from build123d import *

# Parameters (mm, degrees)
SKETCH1_R           = 6
BOSS_EXTRUDE1_DEPTH = 10
BOSS_EXTRUDE1_TAPER = 15
SKETCH2_R           = 2
CUT_EXTRUDE1_DEPTH  = 14.114877049
SKETCH3_W           = 4.267949192
SKETCH3_H           = 2
CUT_EXTRUDE2_DEPTH  = 14.114877049


with BuildPart() as part:
    # Sketch1 → Boss-Extrude1 (new body)
    with BuildSketch(Plane.XY):
        Circle(SKETCH1_R)
    extrude(amount=BOSS_EXTRUDE1_DEPTH, taper=BOSS_EXTRUDE1_TAPER)

    # Sketch2 → Cut-Extrude1 (cut, through all)
    with BuildSketch(Plane(origin=(0, 0, 0), x_dir=(-1, 0, 0), z_dir=(0, 0, -1))):
        Circle(SKETCH2_R)
    extrude(amount=-CUT_EXTRUDE1_DEPTH, mode=Mode.SUBTRACT)

    # Sketch3 → Cut-Extrude2 (cut, through all)
    with BuildSketch(Plane(origin=(0, 0, 0), x_dir=(-1, 0, 0), z_dir=(0, 0, -1))):
        with Locations((-3.866025404, 0)):
            Rectangle(SKETCH3_W, SKETCH3_H)
    extrude(amount=-CUT_EXTRUDE2_DEPTH, mode=Mode.SUBTRACT)


solid = part.part
Could you check a few things on this model? Use its own coordinates, in mm. Round coordinates to 2 decimals unless told otherwise and drop trailing zeros. Write each loop counter-clockwise with the first axis right and the second up, starting at its lowest first coordinate (ties: lowest second). Pieces come first, ordered by that corner, then holes. Notation, with made-up numbers: (81, 70.25) - (140, 70.25) arc R19 ccw to (140, 97.25) - close; hole circle Ø1 at (75.25, 83.25). An arc over 180 degrees is marked (long way). Put each result on its own line as item: value. Start each with the question number.
(1) Will these pins go through, and if not, where does the flat tip stop? pin 1 (1.3 mm diameter, centred on x = 3.5, z = 7, fed in from +Y); pin 2 (3.5 mm diameter, centred on x = 3.5, z = 6, fed in from -Y); pin 3 (4 mm diameter, centred on x = 3, z = 5.5, fed in from -Y); pin 4 (6 mm diameter, centred on x = 1, z = 2, fed in from -Y).
(2) Thinking about a two-plate mould opening in Y: for faces 1 (the flat face through (0, -3, 0)), 2 (the flat face through (3, -1, 4)), 3 (the flat face through (3, 1, 4)), 4 (the conical face through (-4.34, 0.18, 6.18)), which applies, released by +Y, released by -Y, zero draft, split by the parting line, or undercut?
(3) I need wall thicknesses on probe 1 along Y at (x, z) = (0.25, 6); probe 2 along Y at (x, z) = (0.5, 8.75); probe 3 along X at (y, z) = (0, 5.5). Which ranges of each line are inside material? Lowest first, please.
(4) I want a section at C-C, the plane z = 1.5. Please give me the cut outline in (x, y), plus the area to 3 significant figures.
(5) I want a section at B-B, the plane y = 0. Please give me the cut outline in (x, z), plus the area to 3 significant figures.
(6) I want a section at A-A, the plane x = 0. Please give me the cut outline in (y, z), plus the area to 3 significant figures.
Here are the results:
1. pin 1: stops at y = 3.03
1. pin 2: stops at y = -4.18
1. pin 3: stops at y = -4.64
1. pin 4: stops at y = -6
2. face 1: zero draft
2. face 2: undercut
2. face 3: undercut
2. face 4: split by the parting line
3. probe 1: y = -4.39 to -1.98, 1.98 to 4.39
3. probe 2: y = -3.62 to -1.94, 1.94 to 3.62
3. probe 3: x = -4.53 to -2
4. outline: (1.73, -1) arc R2 cw (long way) to (1.73, 1) - (5.51, 1) arc R5.6 ccw (long way) to (5.51, -1) - close
4. area: 78.6 mm^2
5. outline: (-6, 0) - (-2, 0) - (-2, 10) - (-3.32, 10) - close
5. area: 26.6 mm^2
6. outline: (-6, 0) - (-2, 0) - (-2, 10) - (-3.32, 10) - close; (2, 0) - (6, 0) - (3.32, 10) - (2, 10) - close
6. area: 53.2 mm^2
